Here's how the part is built. I have some questions about the finished solid (model axes, mm). Round coordinates to 2 decimals unless told otherwise and drop trailing zeros. Loops run counter-clockwise (first coordinate to the right, second up) from the corner with the lowest first, then second, coordinate; pieces in that order, holes last. Notation, with made-up numbers: M 70.5,23 L 124.5,23 A22 ccw 124.5,32 Z; hole C 14,-8 d4. An arc over 180 degrees is marked long. Use a Markdown table: item, result.
Autodesk Inventor part; units mm, degrees
ref_plane "YZ Plane" through (0, 0, 0) normal (1, 0, 0) x (0, 1, 0)
ref_plane "XZ Plane" through (0, 0, 0) normal (0, 1, 0) x (-1, 0, 0)
ref_plane "XY Plane" through (0, 0, 0) normal (0, 0, 1) x (1, 0, 0)
sketch "Sombreado_1" plane through (0, 0, 0) normal (0, 0, 1) x (1, 0, 0)
  point P0 (0, 0)
sketch "Sombreado_2" plane through (0, 0, 0) normal (0, 0, 1) x (1, 0, 0)
  point P0 (0, 0)
sketch "Sombreado_3" plane through (0, 0, 0) normal (0, 0, 1) x (1, 0, 0)
  point P0 (0, 0)
sketch "Boceto1" plane through (0, 0, 0) normal (0, 1, 0) x (-1, 0, 0)
  line L0 (30.3882, 1.25) -> (30.8882, 1.25)
  line L1 (0, -6.75) -> (75, -6.75)
  line L2 (75, -6.75) -> (75, 18.25)
  line L3 (75, 18.25) -> (0, 18.25)
  line L4 (0, 18.25) -> (0, -6.75)
  arc A0 (21.3882, 1.25) -> (30.8882, 1.25) centre (26.1382, 1.25) ccw
  arc A1 (21.8882, 1.25) -> (30.3882, 1.25) centre (26.1382, 1.25) ccw
  line L5 (21.3882, 1.25) -> (21.8882, 1.25)
  line L6 (1.8, 2.5) -> (5.3, 2.5)
  line L7 (1.8, 2.5) -> (1.8, 3)
  line L8 (1.8, 3) -> (1, 3)
  line L9 (1, 3) -> (1, 2.5)
  line L10 (1, 0) -> (0, 0)
  line L11 (1, 0) -> (1, -0.5)
  line L12 (1, -0.5) -> (1.8, -0.5)
  line L13 (1.8, -0.5) -> (1.8, 0)
  line L14 (5.3, 0) -> (1.8, 0)
  line L15 (0, 2.5) -> (1, 2.5)
  line L16 (1.8, 11.5) -> (5.3, 11.5)
  line L17 (5.3, 9) -> (1.8, 9)
  line L18 (1, 9) -> (0, 9)
  line L19 (0, 11.5) -> (1, 11.5)
  line L20 (1.8, 11.5) -> (1.8, 12)
  line L21 (1.8, 12) -> (1, 12)
  line L22 (1, 12) -> (1, 11.5)
  line L23 (1, 9) -> (1, 8.5)
  line L24 (1, 8.5) -> (1.8, 8.5)
  line L25 (1.8, 8.5) -> (1.8, 9)
  line L26 (44.6082, 1.25) -> (44.1082, 1.25)
  arc A2 (44.1082, 1.25) -> (53.6082, 1.25) centre (48.8582, 1.25) ccw
  arc A3 (44.6082, 1.25) -> (53.1082, 1.25) centre (48.8582, 1.25) ccw
  line L27 (53.6082, 1.25) -> (53.1082, 1.25)
  line L28 (73.1964, 2.5) -> (69.6964, 2.5)
  line L29 (69.6964, 0) -> (73.1964, 0)
  line L30 (73.9964, 0) -> (74.9964, 0)
  line L31 (74.9964, 2.5) -> (73.9964, 2.5)
  line L32 (73.1964, 2.5) -> (73.1964, 3)
  line L33 (73.1964, 3) -> (73.9964, 3)
  line L34 (73.9964, 3) -> (73.9964, 2.5)
  line L35 (73.9964, 0) -> (73.9964, -0.5)
  line L36 (73.9964, -0.5) -> (73.1964, -0.5)
  line L37 (73.1964, -0.5) -> (73.1964, 0)
  line L38 (73.1964, 11.5) -> (69.6964, 11.5)
  line L39 (69.6964, 9) -> (73.1964, 9)
  line L40 (73.9964, 9) -> (74.9964, 9)
  line L41 (74.9964, 11.5) -> (73.9964, 11.5)
  line L42 (73.1964, 11.5) -> (73.1964, 12)
  line L43 (73.1964, 12) -> (73.9964, 12)
  line L44 (73.9964, 12) -> (73.9964, 11.5)
  line L45 (73.9964, 9) -> (73.9964, 8.5)
  line L46 (73.9964, 8.5) -> (73.1964, 8.5)
  line L47 (73.1964, 8.5) -> (73.1964, 9)
  line L48 (75, 18.25) -> (75, 43.25)
  line L49 (75, 43.25) -> (0, 43.25)
  line L50 (0, 43.25) -> (0, 18.25)
  line L51 (5.3, 11.5) -> (5.3, 9)
  line L52 (5.3, 2.5) -> (5.3, 0)
  line L53 (69.6964, 11.5) -> (69.6964, 9)
  line L54 (69.6964, 2.5) -> (69.6964, 0)
  circle A4 centre (26.1382, 1.25) radius 3.25
  circle A5 centre (48.8582, 1.25) radius 3.25
  circle A6 centre (26.1382, 26.25) radius 3.25
  circle A7 centre (48.8582, 26.25) radius 3.25
  line L55 (75, 43.25) -> (75, 68.25)
  line L56 (75, 68.25) -> (0, 68.25)
  line L57 (0, 68.25) -> (0, 43.25)
  circle A8 centre (26.1382, 51.25) radius 3.25
  circle A9 centre (48.8582, 51.25) radius 3.25
  point P0 (0, 0)
sketch "Boceto3" plane through (0, 0, 0) normal (0, 1, 0) x (-1, 0, 0)
  line L0 (0, 0) -> (-75, 0)
  line L1 (-75, 0) -> (-75, -25)
  line L2 (-75, -25) -> (0, -25)
  line L3 (0, -25) -> (0, 0)
  line L4 (0, 0) -> (-75, 0)
  line L5 (-75, 0) -> (-75, -25)
  line L6 (-75, -25) -> (0, -25)
  line L7 (0, -25) -> (0, 0)
  dimension "d4" = 75
  dimension "d5" = 25
  dimension "d6" = 75
  dimension "d7" = 25
extrude "Extrusión1" add sketch "Boceto3" along normal blind 2
sketch "Boceto4" plane through (0, 2, 0) normal (0, 1, 0) x (1, 0, 0)
  circle A0 centre (26.1418, 8) radius 3.25
  line L0 (0, 0) -> (75, 0)
  line L1 (75, 25) -> (0, 25)
  circle A1 centre (48.8582, 8) radius 3.25
extrude "Extrusión2" cut sketch "Boceto4" against normal blind 2
sketch "Boceto5" plane through (0, 2, 0) normal (0, 1, 0) x (1, 0, 0)
  line L0 (30.8908, 8) -> (30.3928, 8)
  line L1 (44.1092, 8) -> (44.6072, 8)
  arc A0 (44.6072, 8) -> (48.8582, 12.251) centre (48.8582, 8) ccw
  arc A1 (44.1092, 8) -> (48.8582, 12.749) centre (48.8582, 8) ccw
  arc A2 (26.1418, 12.251) -> (30.3928, 8) centre (26.1418, 8) ccw
  arc A3 (26.1418, 12.749) -> (30.8908, 8) centre (26.1418, 8) ccw
  line L2 (26.1418, 12.251) -> (48.8582, 12.251)
  line L3 (26.1418, 12.749) -> (48.8582, 12.749)
  point P0 (0, 0)
extrude "Extrusión3" cut sketch "Boceto5" against normal blind 1
properties part number "2ureactor TorusTapa1" material "PPS Plastic"
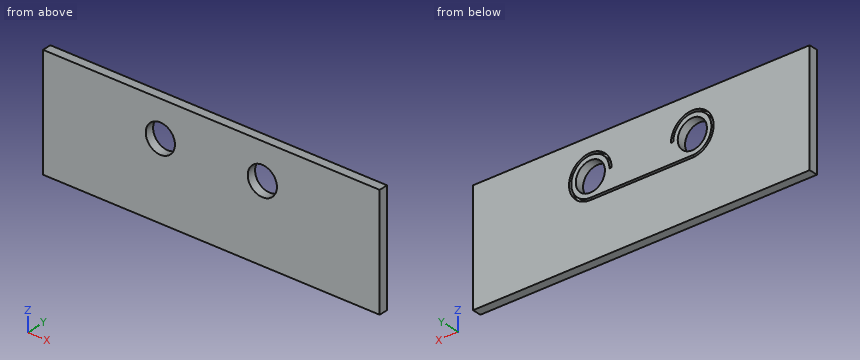
1. I need wall thicknesses on probe 1 along X at (y, z) = (0.95, -8); probe 2 along Z at (x, y) = (49, 1.25); probe 3 along Z at (x, y) = (30, 1.15). Which ranges of each line are inside material? Lowest first, please. Write a range as from..to.
Answer sheet:
| item | result |
|---|---|
| probe 1 | 0..22.89, 29.39..45.61, 52.11..75 |
| probe 2 | -25..-12.75, -12.25..-11.25, -4.75..-3.75, -3.25..0 |
| probe 3 | -25..-12.75, -12.25..-6.22, -5.23..0 |
2. For pin 1 Ø7.5 at (x, z) = (48.86, -8) entering from +Y, with a flat end and sliding along its axis, tell me the tip position at first contact or that it passes through.
Answer sheet:
| item | result |
|---|---|
| pin 1 | y = 2 |
3. Imagine slicing it at B-B, the plane z = -10. Write out the boundary of the cut face in (x, y), then the cut area to 3 significant figures.
Answer sheet:
| item | result |
|---|---|
| outline | M 0,0 L 23.58,0 L 23.58,2 L 22.39,2 L 22.39,1 L 21.83,1 L 21.83,2 L 0,2 Z; M 28.7,0 L 46.3,0 L 46.3,2 L 28.7,2 Z; M 51.42,0 L 75,0 L 75,2 L 53.17,2 L 53.17,1 L 52.61,1 L 52.61,2 L 51.42,2 Z |
| area | 128 mm2 |
4. Imagine slicing it at A-A, the plane y = 1.35. Write out the boundary of the cut face in (x, z), then the cut area to 3 significant figures.
Answer sheet:
| item | result |
|---|---|
| outline | M 0,-25 L 75,-25 L 75,0 L 0,0 Z; hole C 26.14,-8 d6.5; hole M 26.14,-12.75 L 48.86,-12.75 A4.75 ccw long 44.11,-8 L 44.61,-8 A4.25 cw long 48.86,-12.25 L 26.14,-12.25 A4.25 cw long 30.39,-8 L 30.89,-8 A4.75 ccw long Z; hole C 48.86,-8 d6.5 |
| area | 1,780 mm2 |
